```python
from build123d import *

# Parameters (mm, degrees)
SKETCH1_W           = 50
SKETCH1_H           = 250
BOSS_EXTRUDE2_DEPTH = 20
SKETCH1_4_W         = 50
SKETCH1_4_H         = 250
BOSS_EXTRUDE3_DEPTH = 10
SKETCH1_8_R         = 5
CUT_EXTRUDE7_DEPTH  = 20
SKETCH4_W           = 12.5
SKETCH4_H           = 250
SKETCH4_R           = 5
CUT_EXTRUDE8_DEPTH  = 10


with BuildPart() as part:
    # Sketch1 → Boss-Extrude2 (new body)
    with BuildSketch(Plane.XY):
        with Locations((25, 125)):
            Rectangle(SKETCH1_W, SKETCH1_H)
    extrude(amount=BOSS_EXTRUDE2_DEPTH)

    # Sketch1_4 → Boss-Extrude3 (add)
    with BuildSketch(Plane.XY):
        with Locations((25, 125)):
            Rectangle(SKETCH1_4_W, SKETCH1_4_H)
    extrude(amount=BOSS_EXTRUDE3_DEPTH)

    # Sketch1_8 → Cut-Extrude7 (cut)
    with BuildSketch(Plane.XY):
        with Locations((43.75, 187.5)):
            Circle(SKETCH1_8_R)
        with Locations((43.75, 237.5)):
            Circle(SKETCH1_8_R)
        with Locations((43.75, 212.5)):
            Circle(SKETCH1_8_R)
        with Locations((43.75, 162.5)):
            Circle(SKETCH1_8_R)
        with Locations((43.75, 137.5)):
            Circle(SKETCH1_8_R)
        with Locations((43.75, 112.5)):
            Circle(SKETCH1_8_R)
        with Locations((43.75, 87.5)):
            Circle(SKETCH1_8_R)
        with Locations((43.75, 62.5)):
            Circle(SKETCH1_8_R)
        with Locations((43.75, 37.5)):
            Circle(SKETCH1_8_R)
        with Locations((43.75, 12.5)):
            Circle(SKETCH1_8_R)
    extrude(amount=CUT_EXTRUDE7_DEPTH, mode=Mode.SUBTRACT)

    # Sketch4 → Cut-Extrude8 (cut)
    with BuildSketch(Plane.XY.offset(20)):
        with Locations((43.75, 125)):
            Rectangle(SKETCH4_W, SKETCH4_H)
        with Locations((43.75, 12.5)):
            Circle(SKETCH4_R, mode=Mode.SUBTRACT)
        with Locations((43.75, 37.5)):
            Circle(SKETCH4_R, mode=Mode.SUBTRACT)
        with Locations((43.75, 62.5)):
            Circle(SKETCH4_R, mode=Mode.SUBTRACT)
        with Locations((43.75, 87.5)):
            Circle(SKETCH4_R, mode=Mode.SUBTRACT)
        with Locations((43.75, 112.5)):
            Circle(SKETCH4_R, mode=Mode.SUBTRACT)
        with Locations((43.75, 137.5)):
            Circle(SKETCH4_R, mode=Mode.SUBTRACT)
        with Locations((43.75, 162.5)):
            Circle(SKETCH4_R, mode=Mode.SUBTRACT)
        with Locations((43.75, 187.5)):
            Circle(SKETCH4_R, mode=Mode.SUBTRACT)
        with Locations((43.75, 212.5)):
            Circle(SKETCH4_R, mode=Mode.SUBTRACT)
        with Locations((43.75, 237.5)):
            Circle(SKETCH4_R, mode=Mode.SUBTRACT)
    extrude(amount=-CUT_EXTRUDE8_DEPTH, mode=Mode.SUBTRACT)


solid = part.part
```
The listing builds one solid part. Answer for the finished solid, in the listing's coordinates (mm). A direction names the side the tool comes from. Round coordinates to 2 decimals unless told otherwise and drop trailing zeros. Write each loop counter-clockwise with the first axis right and the second up, starting at its lowest first coordinate (ties: lowest second). Pieces come first, ordered by that corner, then holes. Notation, with made-up numbers: (77, 44.25) -> (84, 44.25) arc R11 ccw to (84, 63.25) -> close; hole circle Ø3 at (-5.75, -32.5). An arc over 180 degrees is marked (long way). Use CSV: the item, a comma, the result in double quotes. Start each with the question number.
(1) Each of these flat-tipped pins is pushed along its axis until it touches: pin 1 (13 mm diameter, centred on x = 43.75, y = 212.5, fed in from -Z); pin 2 (5 mm diameter, centred on y = 169.5, z = 17, fed in from +X); pin 3 (4 mm diameter, centred on x = 41.5, y = 127.5, fed in from +Z); pin 4 (6 mm diameter, centred on x = 43.75, y = 237.5, fed in from +Z). Where does it stop, or does it pass through?
(2) Which of the six approach directions +Z, -Z, +X, -X, +Y, -Y give full straight-line access (tool end or side, diameter ignored) to faces 1 (the face through (44, 127, 10)), 2 (the face through (25, 250, 10))?
(3) Section A-A on y = 212.5 is taken. Give the vertices of the cut face in (x, z).
(4) Consider L1, parallel to X at y = 105, z = 18.25; L2, parallel to X at y = 83, z = 4.5; L3, parallel to Z at x = 46.5, y = 128. Determine where each line is inside the solid, lowest interval first. Write a range as from..to.
(5) The mould has two halves that part along Y. Classify faces 3 (the face through (25, 0, 10)), 4 (the face through (39.78, 134.46, 4.93)), 5 (the face through (43.099, 242.457, 4.93)), 6 (the face through (25, 127, 0)): released by +Y, released by -Y, zero draft, split by the parting line, or undercut.
(6) Section D-D on z = 13.75 is taken. Give the vertices of the cut face in (x, y), then the cut area to 4 significant figures.
(7) Section B-B on z = 3 is taken. Count the separate pieces of the cut face and the enclosed holes in it, then the cut area to 3 significant figures.
(8) Section C-C on y = 125.5 is taken. Give the vertices of the cut face in (x, z).
A:
1,pin 1,"stops at z = 0"
1,pin 2,"stops at x = 37.5"
1,pin 3,"stops at z = 10"
1,pin 4,"passes through"
2,face 1,"+Z, +X, +Y, -Y"
2,face 2,"+Z, -Z, +X, -X, +Y"
3,outline,"(0, 0) -> (38.75, 0) -> (38.75, 10) -> (37.5, 10) -> (37.5, 20) -> (0, 20) -> close; (48.75, 0) -> (50, 0) -> (50, 10) -> (48.75, 10) -> close"
4,L1,"x = 0..37.5"
4,L2,"x = 0..41.57, 45.93..50"
4,L3,"z = 0..10"
5,face 3,"released by -Y"
5,face 4,"undercut"
5,face 5,"undercut"
5,face 6,"zero draft"
6,outline,"(0, 0) -> (37.5, 0) -> (37.5, 250) -> (0, 250) -> close"
6,area,"9,375 mm²"
7,separate pieces,"1"
7,enclosed holes,"10"
7,area,"11,700 mm²"
8,outline,"(0, 0) -> (50, 0) -> (50, 10) -> (37.5, 10) -> (37.5, 20) -> (0, 20) -> close"
